```python
from build123d import *

# Parameters (mm, degrees)
SKETCH1_R           = 10
BOSS_EXTRUDE1_DEPTH = 3
SKETCH2_W           = 2
SKETCH2_H           = 3
BOSS_EXTRUDE2_DEPTH = 2
CIRPATTERN1_COUNT   = 3
SKETCH3_R           = 9
SKETCH3_R_2         = 4.5
CUT_EXTRUDE1_DEPTH  = 2
SKETCH4_R           = 1.5
CUT_EXTRUDE2_DEPTH  = 3
BOSS_EXTRUDE3_START = -3
BOSS_EXTRUDE3_DEPTH = 11
CIRPATTERN2_COUNT   = 5


with BuildPart() as part:
    # Sketch1 → Boss-Extrude1 (new body)
    with BuildSketch(Plane(origin=(0, 0, 0), x_dir=(1, 0, 0), z_dir=(0, 1, 0))):
        Circle(SKETCH1_R)
    extrude(amount=BOSS_EXTRUDE1_DEPTH)

    # Sketch2 → Boss-Extrude2 (add)
    with BuildSketch(Plane(origin=(0, 3, 0), x_dir=(1, 0, 0), z_dir=(0, 1, 0))):
        with Locations((0, 4.5)):
            Rectangle(SKETCH2_W, SKETCH2_H)
    boss_extrude2 = extrude(amount=BOSS_EXTRUDE2_DEPTH)

    # CirPattern1: Boss-Extrude2 ×3 about axis
    cirpattern1_axis = Axis((0, 0, 0), (0, 1, 0))
    for i in range(1, CIRPATTERN1_COUNT):
        add(boss_extrude2.rotate(cirpattern1_axis, i * 360 / CIRPATTERN1_COUNT))

    # Sketch3 → Cut-Extrude1 (cut)
    with BuildSketch(Plane(origin=(0, 3, 0), x_dir=(1, 0, 0), z_dir=(0, 1, 0))):
        Circle(SKETCH3_R)
        Circle(SKETCH3_R_2, mode=Mode.SUBTRACT)
    extrude(amount=CUT_EXTRUDE1_DEPTH, mode=Mode.SUBTRACT)

    # Sketch4 → Cut-Extrude2 (cut)
    with BuildSketch(Plane(origin=(0, 3, 0), x_dir=(1, 0, 0), z_dir=(0, 1, 0))):
        Circle(SKETCH4_R)
    extrude(amount=-CUT_EXTRUDE2_DEPTH, mode=Mode.SUBTRACT)

    # Sketch5 → Boss-Extrude3 (add)
    with BuildSketch(Plane(origin=(0, 3, 0), x_dir=(1, 0, 0), z_dir=(0, 1, 0)).offset(BOSS_EXTRUDE3_START)):
        with BuildLine():
            ThreePointArc((3, 11.618950039), (1.51205151, 11.904356355), (0, 12))
            ThreePointArc((0, 12), (-1.51205151, 11.904356355), (-3, 11.618950039))
            Line((-3, 11.618950039), (-3, 9.539392014))
            ThreePointArc((-3, 9.539392014), (0, 10), (3, 9.539392014))
            Line((3, 9.539392014), (3, 11.618950039))
        make_face()
    boss_extrude3 = extrude(amount=BOSS_EXTRUDE3_DEPTH)

    # CirPattern2: Boss-Extrude3 ×5 about axis
    cirpattern2_axis = Axis((0, 0, 0), (0, 1, 0))
    for i in range(1, CIRPATTERN2_COUNT):
        add(boss_extrude3.rotate(cirpattern2_axis, i * 360 / CIRPATTERN2_COUNT))


solid = part.part
```
Here's how the part is built. I have some questions about the finished solid (model axes, mm). A direction names the side the tool comes from. Coordinates: 2 decimals unless noted, no trailing zeros. Order: outer loops, then holes, each group sorted by start corner. A loop starts at its lowest first (then second) coordinate and runs counter-clockwise, first axis right, second up.
Item 1: I need wall thicknesses on probe 1 along X at (y, z) = (0.9, 0); probe 2 along Z at (x, y) = (0, 1.4); probe 3 along Y at (x, z) = (5.5, 5.5). Which ranges of each line are inside material? Lowest first, please.
Response values:
probe 1: x = -10 to -1.5, 1.5 to 10
probe 2: z = -12 to -1.5, 1.5 to 10
probe 3: y = 0 to 3
Item 2: I'm going to push flat-ended pins straight in: pin 1 Ø1.7 at (y, z) = (7, -11) entering from -X; pin 2 Ø0.6 at (x, y) = (0, 4) entering from +Z; pin 3 Ø1.1 at (y, z) = (4, -3.5) entering from -X. Where does each tip first touch, or does it pass through?
Response values:
pin 1: stops at x = -3
pin 2: stops at z = -3
pin 3: stops at x = -11.63
Item 3: Which directions (+Z, -Z, +X, -X, +Y, -Y) give clear straight access to the entire face, cutting with the end or side of a thin tool? Please do faces 1 (the face through (9.496, 1.479, 3.133)), 2 (the face through (3, 5, 2)), 3 (the face through (-3.904, 3.986, 2.238)), 4 (the face through (0, 4, -3)), 5 (the face through (-2.6, 4, 1.5)).
Response values:
face 1: +X, +Y, -Y
face 2: +X, -X, +Y
face 3: -X, +Y
face 4: +Z, +Y
face 5: +Y
Item 4: If we section it at B-B, the plane y = 9.75: List the corners of the cut face in (x, z) for me.
Response values:
outline: (-11.98, -0.74) arc R12 ccw to (-10.12, -6.44) - (-8.15, -5.8) arc R10 cw to (-10, -0.09) - close; (-9.26, 7.64) - (-8.03, 5.95) arc R10 cw to (-3.18, 9.48) - (-4.4, 11.16) arc R12 ccw to start; (-3, -11.62) arc R12 ccw to (3, -11.62) - (3, -9.54) arc R10 cw to (-3, -9.54) - close; (3.18, 9.48) arc R10 cw to (8.03, 5.95) - (9.26, 7.64) arc R12 ccw to (4.4, 11.16) - close; (8.15, -5.8) - (10.12, -6.44) arc R12 ccw to (11.98, -0.74) - (10, -0.09) arc R10 cw to start
Item 5: If we section it at A-A, the plane y = 2.25: List the corners of the cut face in (x, z) for me, then the cut area to 3 significant figures.
Response values:
outline: (-11.98, -0.74) arc R12 ccw to (-10.12, -6.44) - (-8.15, -5.8) arc R10 ccw to (-3, -9.54) - (-3, -11.62) arc R12 ccw to (3, -11.62) - (3, -9.54) arc R10 ccw to (8.15, -5.8) - (10.12, -6.44) arc R12 ccw to (11.98, -0.74) - (10, -0.09) arc R10 ccw to (8.03, 5.95) - (9.26, 7.64) arc R12 ccw to (4.4, 11.16) - (3.18, 9.48) arc R10 ccw to (-3.18, 9.48) - (-4.4, 11.16) arc R12 ccw to (-9.26, 7.64) - (-8.03, 5.95) arc R10 ccw to (-10, -0.09) - close; hole circle Ø3 at (0, 0)
area: 368 mm2
Item 6: If we section it at D-D, the plane z = -6.75: List the corners of the cut face in (x, y) for me.
Response values:
outline: (-7.38, 0) - (7.38, 0) - (7.38, 3) - (-7.38, 3) - close
Item 7: Thinking about a two-plate mould opening in X: for faces 6 (the face through (-3.69, 3.986, 0.976)), 7 (the face through (2.69, 3.99, 2.71)), 8 (the face through (-3, 5, 2)), 9 (the face through (8.654, 5.423, 6.807)), which applies, pulls with the +X half, pulls with the -X half, needs draft (parallel to the pull), parting line crosses it, or undercut?
Response values:
face 6: pulls with the -X half
face 7: undercut
face 8: needs draft
face 9: pulls with the +X half
Item 8: If we section it at C-C, the plane y = 4.5: Give the number of separate pieces and of enclosed holes in the cut face, then the cut area to 3 significant figures.
Response values:
separate pieces: 8
enclosed holes: 0
area: 69.6 mm2
